from build123d import *

# Parameters (mm, degrees)
F0_R     = 10.85
F1_DEPTH = 8


with BuildPart() as f1:
    # F0 (on Top) → F1 (new body)
    with BuildSketch(Plane.XY):
        with BuildLine():
            Line((9.131195, 24.862669), (9.131195, 39.862669))
            ThreePointArc((9.131195, 39.862669), (11.903994, 51.842548), (1.839538, 58.907434))
            Line((1.839538, 58.907434), (2.025343, 55.758941))
            Line((2.025343, 55.758941), (1.158253, 55.745472))
            Line((1.158253, 55.745472), (1.158253, 58.899236))
            ThreePointArc((1.158253, 58.899236), (-8.688188, 51.71865), (-5.868805, 39.862669))
            Line((-5.868805, 39.862669), (-5.868805, 24.862669))
            ThreePointArc((-5.868805, 24.862669), (-14.4659, 19.970502), (-14.65131, 10.080661))
            ThreePointArc((-14.65131, 10.080661), (-25.307738, 6.64516), (-26.0973, -4.523488))
            Line((-26.0973, -4.523488), (-39.087681, -12.023488))
            ThreePointArc((-39.087681, -12.023488), (-50.84896, -15.612113), (-51.935103, -27.860631))
            Line((-51.935103, -27.860631), (-49.301331, -26.125472))
            Line((-49.301331, -26.125472), (-48.856122, -26.86966))
            Line((-48.856122, -26.86966), (-51.587361, -28.446542))
            ThreePointArc((-51.587361, -28.446542), (-40.445571, -33.383517), (-31.587681, -25.013869))
            Line((-31.587681, -25.013869), (-18.5973, -17.513869))
            ThreePointArc((-18.5973, -17.513869), (-10.062012, -22.513088), (-1.404453, -17.728738))
            ThreePointArc((-1.404453, -17.728738), (6.898991, -25.239724), (16.966106, -20.339181))
            Line((16.966106, -20.339181), (29.956487, -27.839181))
            ThreePointArc((29.956487, -27.839181), (38.944966, -36.230435), (50.095566, -31.046804))
            Line((50.095566, -31.046804), (47.275988, -29.633469))
            Line((47.275988, -29.633469), (47.697869, -28.875812))
            Line((47.697869, -28.875812), (50.429108, -30.452694))
            ThreePointArc((50.429108, -30.452694), (49.133759, -18.335133), (37.456487, -14.8488))
            Line((37.456487, -14.8488), (24.466106, -7.3488))
            ThreePointArc((24.466106, -7.3488), (24.527912, 2.542586), (16.055764, 7.648077))
            ThreePointArc((16.055764, 7.648077), (18.408746, 18.594564), (9.131195, 24.862669))
        make_face()
        Circle(F0_R, mode=Mode.SUBTRACT)
    extrude(amount=F1_DEPTH)


solid = f1.part
For this review, take the finished solid that the model builds, in its own axes (mm). A direction names the side the tool comes from. Give positions to 0.01 mm unless a question says otherwise; leave off trailing zeros. Loops run counter-clockwise (first coordinate to the right, second up) from the corner with the lowest first, then second, coordinate; pieces in that order, holes last.
Item 1: Tool access review of faces 4 (the flat face through (9.131, 32, 4)), 5 (the flat face through (-50.203, -27.647, 3.944)), 6 (the flat face through (-5.869, 32, 4)), 7 (the flat face through (1.158, 57, 4)): name each direction out of +Z, -Z, +X, -X, +Y, -Y from which nothing blocks a thin tool from reaching the whole face with its end or side.
Item 2: Take a section at C-C, the plane z = 6.75. State the section outline as (x, y) points.
Item 3: Draft analysis for pull direction X (two halves, no side actions). For faces 1 (the cylindrical face through (-8.624, 51.888, 3.944)), 2 (the cylindrical face through (38.76, -36.2, 3.94)), 3 (the flat face through (-5, -10, 8)), state which applies: +X half, -X half, draft (parallel to the pull), parting line (faces both ways), or undercut.
Item 4: Insertion check: pin 1 (0.9 mm diameter, centred on y = 57, z = 2.5, fed in from +X); pin 2 (2.5 mm diameter, centred on y = 32, z = 5, fed in from +X); pin 3 (4 mm diameter, centred on x = 37.5, z = 2.5, fed in from +Y); pin 4 (25 mm diameter, centred on x = 0, y = 0, fed in from +Z). Each pin has a flat end and moves straight along its axis. Give the tip position at first contact, or say it passes through.
Item 5: Take a section at A-A, the plane x = 0. State the section outline as (y, z) points, and give its area (3 significant figures).
Item 6: Take a section at B-B, the plane y = 0. State the section outline as (x, z) points.
Item 7: Take a section at D-D, the plane y = 38. State the section outline as (x, z) points, and give its area (3 significant figures).
Item 8: For line 1 along X through (y, z) = (31, 4); line 2 along Y through (x, z) = (0, 2.75); line 3 along X through (y, z) = (-8.5, 5), list the stretches that pass through material, from the lowest coordinate up.
Calculated:
1. face 4: +Z, -Z, +X
1. face 5: +Z, -Z
1. face 6: +Z, -Z, -X
1. face 7: +Z, -Z, +Y
2. outline: (-51.94, -27.86) - (-49.3, -26.13) - (-48.86, -26.87) - (-51.59, -28.45) arc R11 ccw to (-31.59, -25.01) - (-18.6, -17.51) arc R10 ccw to (-1.4, -17.73) arc R10 ccw to (16.97, -20.34) - (29.96, -27.84) arc R11 ccw to (50.1, -31.05) - (47.28, -29.63) - (47.7, -28.88) - (50.43, -30.45) arc R11 ccw to (37.46, -14.85) - (24.47, -7.35) arc R10 ccw to (16.06, 7.65) arc R10 ccw to (9.13, 24.86) - (9.13, 39.86) arc R11 ccw to (1.84, 58.91) - (2.03, 55.76) - (1.16, 55.75) - (1.16, 58.9) arc R11 ccw to (-5.87, 39.86) - (-5.87, 24.86) arc R10 ccw to (-14.65, 10.08) arc R10 ccw to (-26.1, -4.52) - (-39.09, -12.02) arc R11 ccw to start; hole circle Ø21.7 at (0, 0)
3. face 1: -X half
3. face 2: undercut
3. face 3: draft
4. pin 1: stops at x = 8.44
4. pin 2: stops at x = 9.13
4. pin 3: stops at y = -13.72
4. pin 4: stops at z = 8
5. outline: (-20.91, 0) - (-10.85, 0) - (-10.85, 8) - (-20.91, 8) - close; (10.85, 0) - (58.79, 0) - (58.79, 8) - (10.85, 8) - close
5. area: 464 mm2
6. outline: (-27.43, 0) - (-10.85, 0) - (-10.85, 8) - (-27.43, 8) - close; (10.85, 0) - (25.53, 0) - (25.53, 8) - (10.85, 8) - close
7. outline: (-5.87, 0) - (9.13, 0) - (9.13, 8) - (-5.87, 8) - close
7. area: 120 mm2
8. line 1: x = -5.87 to 9.13
8. line 2: y = -20.91 to -10.85, 10.85 to 58.79
8. line 3: x = -32.98 to -6.74, 6.74 to 26.46
